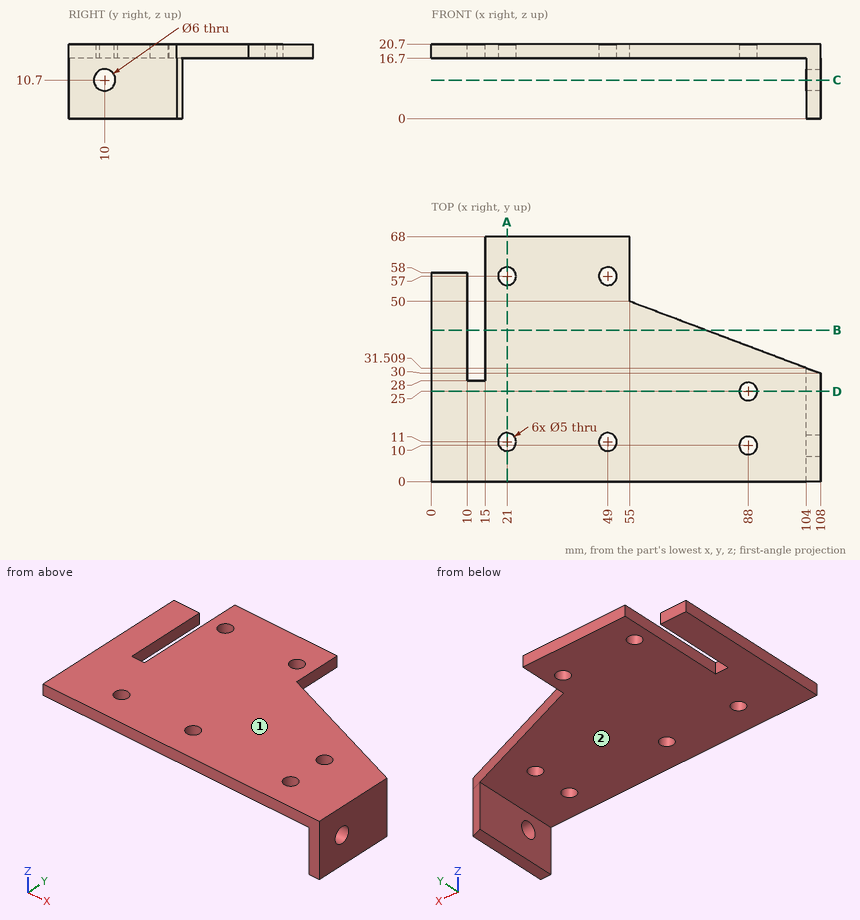
Here's the drawing with two shaded views (mm, measured from the low corner). I have some questions. A direction names the side the tool comes from. Round coordinates to 2 decimals unless told otherwise and drop trailing zeros. Order: outer loops, then holes, each group sorted by start corner. A loop starts at its lowest first (then second) coordinate and runs counter-clockwise, first axis right, second up. Notation, with made-up numbers: (21.25, 37) -> (78.25, 37) arc R23 ccw to (78.25, 73) -> close; hole circle Ø5 at (80, 58). An arc over 180 degrees is marked (long way). Use a Markdown table: item, result. Add a question column.
(1) Suppose I cut it at A-A, the plane x = 21. Please give me the cut outline in (y, z).
(2) Suppose I cut it at B-B, the plane y = 42. Please give me the cut outline in (x, z).
(3) For pin 1 Ø4 at (x, y) = (88, 25) entering from +Z; pin 2 Ø2 at (y, z) = (60.5, 19.5) entering from +X; pin 3 Ø6 at (x, y) = (49, 11) entering from -Z; pin 4 Ø4.5 at (x, z) = (6, 18) entering from +Y, each with a flat end and sliding along its axis, tell me the tip position at first contact or that it passes through.
(4) I need wall thicknesses on line 1 along Y through (x, z) = (49, 19.3); line 2 along X through (y, z) = (54, 19); line 3 along Z through (x, y) = (32, 60). Which ranges of each line are inside material? Lowest first, please.
(5) Suppose I cut it at D-D, the plane y = 25. Please give me the cut outline in (x, z), and give its area (3 significant figures).
(6) For the marked faces 1 and 2, which set-ups out of +Z, -Z, +X, -X, +Y, -Y let a thin tool reach every point of the face, with its end or its side?
(7) Suppose I cut it at C-C, the plane z = 10.7. Please give me the cut outline in (x, y).
Verdict:
| question | item | result |
|---|---|---|
| 1 | outline | (0, 16.7) -> (8.5, 16.7) -> (8.5, 20.7) -> (0, 20.7) -> close; (13.5, 16.7) -> (54.5, 16.7) -> (54.5, 20.7) -> (13.5, 20.7) -> close; (59.5, 16.7) -> (68, 16.7) -> (68, 20.7) -> (59.5, 20.7) -> close |
| 2 | outline | (0, 16.7) -> (10, 16.7) -> (10, 20.7) -> (0, 20.7) -> close; (15, 16.7) -> (76.2, 16.7) -> (76.2, 20.7) -> (15, 20.7) -> close |
| 3 | pin 1 | through |
| 3 | pin 2 | x = 55 |
| 3 | pin 3 | z = 16.7 |
| 3 | pin 4 | y = 58 |
| 4 | line 1 | 0 to 8.5, 13.5 to 54.5, 59.5 to 68 |
| 4 | line 2 | 0 to 10, 15 to 55 |
| 4 | line 3 | 16.7 to 20.7 |
| 5 | outline | (0, 16.7) -> (85.5, 16.7) -> (85.5, 20.7) -> (0, 20.7) -> close; (90.5, 16.7) -> (104, 16.7) -> (104, 0) -> (108, 0) -> (108, 20.7) -> (90.5, 20.7) -> close |
| 5 | area | 479 mm2 |
| 6 | face 1 | +Z, +X, -X, +Y, -Y |
| 6 | face 2 | -Z, -X, +Y, -Y |
| 7 | outline | (104, 0) -> (108, 0) -> (108, 7) -> (104, 7) -> close; (104, 13) -> (108, 13) -> (108, 30) -> (104, 31.51) -> close |
